```python
from build123d import *

# Parameters (mm, degrees)
BOSS_EXTRUDE1_DEPTH      = 5.08
CUT_EXTRUDE2_START       = -6.0800001
CUT_EXTRUDE2_DEPTH       = 7.0800002
BOSS_EXTRUDE2_DEPTH      = 3.175
SKETCH6_R                = 2.54
BOSS_EXTRUDE3_DEPTH      = 15.24
SKETCH7_R                = 1.524
CUT_EXTRUDE3_DEPTH       = 25.4
CUT_EXTRUDE4_DEPTH       = 5.08
SKETCH9_R                = 0.889
BOSS_EXTRUDE4_DEPTH      = 6.35
FILLET1_R                = 1.27
REVOLVE1_ANGLE           = 7
REVOLVE1_OTHER_WAY_ANGLE = 7


with BuildPart() as part:
    # Sketch2 → Boss-Extrude1 (new body)
    with BuildSketch(Plane.XY):
        with BuildLine():
            ThreePointArc((642.510849283, -1.582039112), (643.111845681, -1.408373102), (643.599082689, -1.016))
            ThreePointArc((643.599082689, -1.016), (642.269121423, -1.135922533), (641.567082689, 0))
            Line((641.567082689, 0), (473.360965279, 0))
            Line((473.360965279, 0), (460.660965279, 0))
            Line((460.660965279, 0), (114.935, 0))
            ThreePointArc((114.935, 0), (104.14, -10.795), (93.345, 0))
            Line((93.345, 0), (53.34, 0))
            ThreePointArc((53.34, 0), (40.64, -12.7), (27.94, 0))
            Line((27.94, 0), (0, 0))
            add(Edge.make_bspline(
                [(0, 0), (0, -1.007496172), (0.154611582, -3.513796615), (1.106333228, -7.923389435), (3.463136343, -13.420354421), (7.689616489, -19.513207632), (13.932423524, -25.726412106), (22.129107375, -31.731455339), (32.141645239, -37.332204029), (43.82045433, -42.41500246), (57.023709725, -46.912543066), (71.619696083, -50.784752003), (87.485018636, -54.008935199), (104.502313427, -56.574303932), (122.558104573, -58.481758104), (141.542033828, -59.739895824), (161.345829027, -60.366961324), (181.863132616, -60.387506142), (202.989192599, -59.8341217), (224.620860897, -58.745176641), (246.65655865, -57.164603829), (268.996310773, -55.141201012), (291.541767704, -52.727712704), (314.196207315, -49.979843895), (336.86454415, -46.955447457), (359.453314895, -43.713502532), (381.870662856, -40.313266856), (404.02631566, -36.813220545), (425.831595832, -33.270324121), (447.199424328, -29.739007432), (468.044367735, -26.27043606), (488.282710288, -22.911672601), (507.832591566, -19.705111663), (526.614143658, -16.687720753), (544.549749946, -13.890665375), (561.564270734, -11.338919625), (577.585454095, -9.050636147), (592.543922516, -7.037634907), (606.374988512, -5.304428983), (619.014124193, -3.849253664), (630.413817462, -2.663385493), (638.093728429, -1.953546407), (641.993392355, -1.625070631), (642.510849283, -1.582039112)],
                knots=[0.5, 0.5, 0.5, 0.5, 0.502166769, 0.505390167, 0.509655974, 0.514947682, 0.521244711, 0.528520886, 0.536744945, 0.54588136, 0.555890751, 0.566730119, 0.57835299, 0.590709588, 0.603747039, 0.617409572, 0.631638768, 0.646373793, 0.661551658, 0.677107483, 0.692974771, 0.709085713, 0.725371443, 0.741762353, 0.758188398, 0.774579367, 0.790865214, 0.806976332, 0.822843867, 0.838400002, 0.853578262, 0.868313774, 0.882543568, 0.896206835, 0.909245173, 0.92160287, 0.933227116, 0.944068236, 0.954079898, 0.963219316, 0.971447445, 0.978729112, 0.979842958, 0.979842958, 0.979842958, 0.979842958], degree=3))
        make_face()
    boss_extrude1 = extrude(amount=BOSS_EXTRUDE1_DEPTH)

    # Sketch3 → Cut-Extrude2 (cut)
    with BuildSketch(Plane.XY.offset(5.08).offset(CUT_EXTRUDE2_START)):
        with BuildLine():
            ThreePointArc((212.767950148, 0), (169.566475074, 43.201475074), (126.365, 0))
            Line((126.365, 0), (212.767950148, 0))
        make_face()
        with BuildLine():
            Line((212.767950148, 0), (126.365, 0))
            ThreePointArc((126.365, 0), (169.566475074, -43.201475074), (212.767950148, 0))
        make_face()
        with BuildLine():
            ThreePointArc((300.809151759, 0), (262.503550953, 38.305600806), (224.197950148, 0))
            Line((224.197950148, 0), (300.809151759, 0))
        make_face()
        with BuildLine():
            Line((300.809151759, 0), (224.197950148, 0))
            ThreePointArc((224.197950148, 0), (262.503550953, -38.305600806), (300.809151759, 0))
        make_face()
        with BuildLine():
            ThreePointArc((369.720663748, 0), (340.979907754, 28.740755995), (312.239151759, 0))
            Line((312.239151759, 0), (369.720663748, 0))
        make_face()
        with BuildLine():
            Line((369.720663748, 0), (312.239151759, 0))
            ThreePointArc((312.239151759, 0), (340.979907754, -28.740755995), (369.720663748, 0))
        make_face()
        with BuildLine():
            ThreePointArc((381.150663748, 0), (400.327663748, -19.177), (419.504663748, 0))
            Line((419.504663748, 0), (381.150663748, 0))
        make_face()
        with BuildLine():
            Line((381.150663748, 0), (419.504663748, 0))
            ThreePointArc((419.504663748, 0), (400.327663748, 19.177), (381.150663748, 0))
        make_face()
        with BuildLine():
            ThreePointArc((430.474866123, 0), (443.301866123, -12.827), (456.128866123, 0))
            Line((456.128866123, 0), (430.474866123, 0))
        make_face()
        with BuildLine():
            Line((430.474866123, 0), (456.128866123, 0))
            ThreePointArc((456.128866123, 0), (443.301866123, 12.827), (430.474866123, 0))
        make_face()
        with BuildLine():
            ThreePointArc((475.605534569, 0), (482.082534569, -6.477), (488.559534569, 0))
            Line((488.559534569, 0), (475.605534569, 0))
        make_face()
        with BuildLine():
            Line((475.605534569, 0), (488.559534569, 0))
            ThreePointArc((488.559534569, 0), (482.082534569, 6.477), (475.605534569, 0))
        make_face()
    cut_extrude2 = extrude(amount=CUT_EXTRUDE2_DEPTH, mode=Mode.SUBTRACT)

    # Mirror1: Boss-Extrude1, Cut-Extrude2 across plane
    add(boss_extrude1.mirror(Plane.ZX))
    add(cut_extrude2.mirror(Plane.ZX), mode=Mode.SUBTRACT)

    # Sketch5 → Boss-Extrude2 (add)
    with BuildSketch(Plane.XY.offset(5.08)):
        with BuildLine():
            Line((640.969745334, -1.721816251), (617.648537938, -3.837034781))
            Line((617.648537938, -3.837034781), (544.313686995, -10.488458656))
            ThreePointArc((544.313686995, -10.488458656), (541.770845349, -8.368527507), (543.890776497, -5.825685861))
            Line((543.890776497, -5.825685861), (608.121505485, 0))
            Line((608.121505485, 0), (543.890776497, 5.825685861))
            ThreePointArc((543.890776497, 5.825685861), (541.770845349, 8.368527507), (544.313686995, 10.488458656))
            Line((544.313686995, 10.488458656), (617.648537938, 3.837034781))
            Line((617.648537938, 3.837034781), (640.969745334, 1.721816251))
            ThreePointArc((640.969745334, 1.721816251), (645.377082689, 0), (640.969745334, -1.721816251))
        make_face()
    extrude(amount=BOSS_EXTRUDE2_DEPTH)

    # Sketch6 → Boss-Extrude3 (add, symmetric)
    with BuildSketch(Plane.XY.offset(8.255)):
        with Locations((642.837082689, 0)):
            Circle(SKETCH6_R)
    extrude(amount=BOSS_EXTRUDE3_DEPTH, both=True)

    # Sketch7 → Cut-Extrude3 (cut)
    with BuildSketch(Plane.XY.offset(23.495)):
        with Locations((642.837082689, 0)):
            Circle(SKETCH7_R)
    extrude(amount=-CUT_EXTRUDE3_DEPTH, mode=Mode.SUBTRACT)

    # Sketch8 → Cut-Extrude4 (cut)
    with BuildSketch(Plane(origin=(0, 0, 0), x_dir=(-1, 0, 0), z_dir=(0, 0, -1))):
        with BuildLine():
            ThreePointArc((-640.961258409, -1.712566282), (-640.297082689, 0), (-640.961258409, 1.712566282))
            add(Edge.make_bspline(
                [(-640.961258409, -1.712566282), (-640.960510251, -1.712630108), (-637.579890575, -2.001039431), (-630.413817462, -2.663385493), (-619.014124193, -3.849253664), (-606.374988512, -5.304428983), (-592.543922516, -7.037634907), (-577.585454095, -9.050636147), (-561.564270734, -11.338919625), (-544.549749946, -13.890665375), (-526.614143658, -16.687720753), (-507.832591566, -19.705111663), (-488.282710288, -22.911672601), (-468.044367735, -26.27043606), (-447.199424328, -29.739007432), (-425.831595832, -33.270324121), (-404.02631566, -36.813220545), (-381.870662856, -40.313266856), (-359.453314895, -43.713502532), (-336.86454415, -46.955447457), (-314.196207315, -49.979843895), (-291.541767704, -52.727712704), (-268.996310773, -55.141201012), (-246.65655865, -57.164603829), (-224.620860897, -58.745176641), (-202.989192599, -59.8341217), (-181.863132616, -60.387506142), (-161.345829027, -60.366961324), (-141.542033828, -59.739895824), (-122.558104573, -58.481758104), (-104.502313427, -56.574303932), (-87.485018636, -54.008935199), (-71.619696083, -50.784752003), (-57.023709725, -46.912543066), (-43.82045433, -42.41500246), (-32.141645239, -37.332204029), (-22.129107375, -31.731455339), (-13.932423524, -25.726412106), (-7.689616489, -19.513207632), (-3.463136343, -13.420354421), (-1.106333228, -7.923389435), (-0.154611582, -3.513796615), (0.062151598, 0), (-0.154611582, 3.513796615), (-1.106333228, 7.923389435), (-3.463136343, 13.420354421), (-7.689616489, 19.513207632), (-13.932423524, 25.726412106), (-22.129107375, 31.731455339), (-32.141645239, 37.332204029), (-43.82045433, 42.41500246), (-57.023709725, 46.912543066), (-71.619696083, 50.784752003), (-87.485018636, 54.008935199), (-104.502313427, 56.574303932), (-122.558104573, 58.481758104), (-141.542033828, 59.739895824), (-161.345829027, 60.366961324), (-181.863132616, 60.387506142), (-202.989192599, 59.8341217), (-224.620860897, 58.745176641), (-246.65655865, 57.164603829), (-268.996310773, 55.141201012), (-291.541767704, 52.727712704), (-314.196207315, 49.979843895), (-336.86454415, 46.955447457), (-359.453314895, 43.713502532), (-381.870662856, 40.313266856), (-404.02631566, 36.813220545), (-425.831595832, 33.270324121), (-447.199424328, 29.739007432), (-468.044367735, 26.27043606), (-488.282710288, 22.911672601), (-507.832591566, 19.705111663), (-526.614143658, 16.687720753), (-544.549749946, 13.890665375), (-561.564270734, 11.338919625), (-577.585454095, 9.050636147), (-592.543922516, 7.037634907), (-606.374988512, 5.304428983), (-619.014124193, 3.849253664), (-630.413817462, 2.663385493), (-637.579890575, 2.001039431), (-640.960510251, 1.712630108), (-640.961258409, 1.712566282)],
                knots=[0.021269276, 0.021269276, 0.021269276, 0.021269276, 0.021270888, 0.028552555, 0.036780684, 0.045920102, 0.055931764, 0.066772884, 0.07839713, 0.090754827, 0.103793165, 0.117456432, 0.131686226, 0.146421738, 0.161599998, 0.177156133, 0.193023668, 0.209134786, 0.225420633, 0.241811602, 0.258237647, 0.274628557, 0.290914287, 0.307025229, 0.322892517, 0.338448342, 0.353626207, 0.368361232, 0.382590428, 0.396252961, 0.409290412, 0.42164701, 0.433269881, 0.444109249, 0.45411864, 0.463255055, 0.471479114, 0.478755289, 0.485052318, 0.490344026, 0.494609833, 0.497833231, 0.5, 0.502166769, 0.505390167, 0.509655974, 0.514947682, 0.521244711, 0.528520886, 0.536744945, 0.54588136, 0.555890751, 0.566730119, 0.57835299, 0.590709588, 0.603747039, 0.617409572, 0.631638768, 0.646373793, 0.661551658, 0.677107483, 0.692974771, 0.709085713, 0.725371443, 0.741762353, 0.758188398, 0.774579367, 0.790865214, 0.806976332, 0.822843867, 0.838400002, 0.853578262, 0.868313774, 0.882543568, 0.896206835, 0.909245173, 0.92160287, 0.933227116, 0.944068236, 0.954079898, 0.963219316, 0.971447445, 0.978729112, 0.978730724, 0.978730724, 0.978730724, 0.978730724], degree=3))
        make_face()
    extrude(amount=-CUT_EXTRUDE4_DEPTH, mode=Mode.SUBTRACT)

    # Sketch9 → Boss-Extrude4 (add)
    with BuildSketch(Plane(origin=(0, 0, 5.08), x_dir=(-1, 0, 0), z_dir=(0, 0, -1))):
        with Locations((-544.102231746, 8.157072259)):
            Circle(SKETCH9_R)
        with Locations((-544.102231746, -8.157072259)):
            Circle(SKETCH9_R)
        with Locations((-580.769657218, 4.831360321)):
            Circle(SKETCH9_R)
        with Locations((-580.769657218, -4.831360321)):
            Circle(SKETCH9_R)
        with Locations((-617.437082689, 0)):
            Circle(SKETCH9_R)
        with Locations((-635.217082689, 0)):
            Circle(SKETCH9_R)
    extrude(amount=BOSS_EXTRUDE4_DEPTH)

    # Fillet1
    fillet1_edges = [part.edges().sort_by_distance(p)[0] for p in [
        (608.121505485, 0, 6.6675),
    ]]
    fillet(fillet1_edges, radius=FILLET1_R)

    # Sketch10 → Revolve1 (revolve)
    with BuildSketch(Plane(origin=(0, 0, 0), x_dir=(1, 0, 0), z_dir=(0, 1, 0))):
        Polygon((640.297082689, -23.495), (598.425526817, -8.255), (640.297082689, -8.255), align=None)
    revolve(axis=Axis((642.837082689, 0, -1.905), (0, 0, 1)), revolution_arc=REVOLVE1_ANGLE)

    # Sketch10 → Revolve1 other way (revolve)
    with BuildSketch(Plane(origin=(0, 0, 0), x_dir=(1, 0, 0), z_dir=(0, 1, 0))):
        Polygon((640.297082689, -23.495), (598.425526817, -8.255), (640.297082689, -8.255), align=None)
    revolve(axis=Axis((642.837082689, 0, -1.905), (0, 0, -1)), revolution_arc=REVOLVE1_OTHER_WAY_ANGLE)


solid = part.part
```
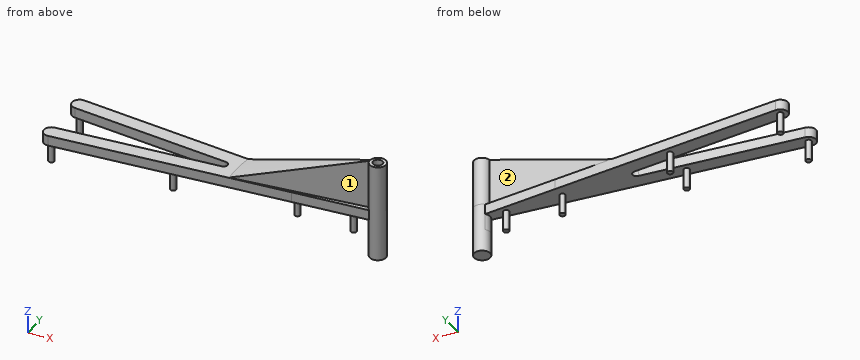
Design review of the part built by this model. Coordinates are the model's own, in mm. Face numbers are marked on the shaded views. A direction names the side the tool comes from. Round coordinates to 2 decimals unless told otherwise and drop trailing zeros. Write each loop counter-clockwise with the first axis right and the second up, starting at its lowest first coordinate (ties: lowest second). Pieces come first, ordered by that corner, then holes. Notation, with made-up numbers: (40.5, -32.75) -> (47.5, -32.75) arc R31 ccw to (47.5, -0.75) -> close; hole circle Ø10 at (-2, 25). An arc over 180 degrees is marked (long way). Write item = value, one per line. Start each with the question number.
1) Take a section at B-B, the plane x = 588.5. State the section outline as (y, z) points (3 decimals), plus the area to 3 significant figures.
2) Wall thickness on probe 1 along Z at (x, y) = (567.5, -7.25) (3 decimals); probe 2 along Y at (x, z) = (617.5, 8); probe 3 along Y at (x, z) = (635.5, 13): over which ranges is each line inside the solid? List them lowest first. Write a range as from..to.
3) Clearance check with flat-ended pins moving along their axes: pin 1 (2.5 mm diameter, centred on x = 642.5, y = 0, fed in from +Z) (3 decimals); pin 2 (1.4 mm diameter, centred on x = 544.5, y = -8, fed in from -Z); pin 3 (10.5 mm diameter, centred on x = 574, y = 4.5, fed in from -Z); pin 4 (6.5 mm diameter, centred on x = 578.5, y = -3.5, fed in from +Z) (3 decimals). State where each tip first meets the part, or that it passes through.
4) Take a section at A-A, the plane z = 3.5. State the section outline as (x, y) points, plus the area to 3 significant figures.
5) Tool access review of the marked faces 1 and 2: name each direction out of +Z, -Z, +X, -X, +Y, -Y from which nothing blocks a thin tool from reaching the whole face with its end or side.
Results list:
q1.outline = (-6.481, 5.08) -> (-1.78, 5.08) -> (-1.78, 8.255) -> (-6.481, 8.255) -> close; (1.78, 5.08) -> (6.481, 5.08) -> (6.481, 8.255) -> (1.78, 8.255) -> close
q1.area = 29.9 mm²
q2.probe_1 = 5.08..8.255
q2.probe_2 = -3.85..3.85
q2.probe_3 = -0.9..0.9
q3.pin_1 = 23.495
q3.pin_2 = -1.27
q3.pin_3 = 5.08
q3.pin_4 = 8.255
q4.outline = circle Ø1.78 at (544.1, -8.16); circle Ø1.78 at (544.1, 8.16); circle Ø1.78 at (580.77, -4.83); circle Ø1.78 at (580.77, 4.83); circle Ø1.78 at (617.44, 0); circle Ø1.78 at (635.22, 0); circle Ø5.08 at (642.84, 0); hole circle Ø3.05 at (642.84, 0)
q4.area = 27.9 mm²
q5.face_1 = +Z, -Y
q5.face_2 = +Z, +Y
